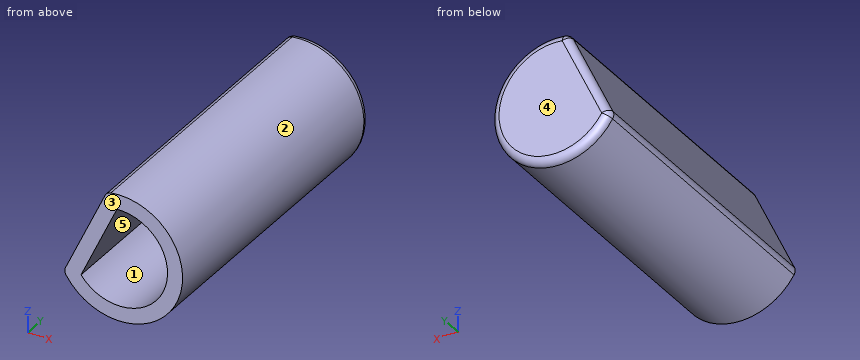
Autodesk Inventor part; units mm, degrees
ref_plane "YZ Plane" through (0, 0, 0) normal (1, 0, 0) x (0, 1, 0)
ref_plane "XZ Plane" through (0, 0, 0) normal (0, 1, 0) x (-1, 0, 0)
ref_plane "XY Plane" through (0, 0, 0) normal (0, 0, 1) x (1, 0, 0)
sketch "Sketch1" plane through (0, 0, 0) normal (0, 1, 0) x (-1, 0, 0)
  arc A0 (0.8395, 4.1153) -> (3.6921, -2.0022) centre (0, 0) ccw
  line L0 (0, -7.6704) -> (0, 6.9519)
  line L1 (-7.5059, 0) -> (5.9652, 0)
  line L2 (3.6921, -2.0022) -> (0.8395, 4.1153)
  dimension "d2" = 8.4
  dimension "d3" = 2.5
  dimension "d4" = 25
extrude "Extrusion1" add sketch "Sketch1" along normal blind 20.4
shell "Shell1" thickness 1 removed faces 1 at (-0.173, 0, 1.1178)
fillet "Fillet1" radius 0.5 2 edges at (-2.2658, 20.4, 1.0565) (3.8065, 20.4, -1.775)
fillet "Fillet2" radius 0.5 4 edges at (-3.5246, 20.2564, -1.9963) (-0.7363, 20.2564, 3.9832) (-0.8395, 9.95, 4.1153) (-3.6921, 9.95, -2.0022)
properties part number "Poti_Verlaengerung"
Can you work these out from the model? Positions are in its coordinate system, mm. Face numbers are marked on the shaded views. A direction names the side the tool comes from. Coordinates: 2 decimals unless noted, no trailing zeros. Loops run counter-clockwise (first coordinate to the right, second up) from the corner with the lowest first, then second, coordinate; pieces in that order, holes last.
Item 1: Please list where these lines run through material, in increasing order: L1, parallel to Z at x = 0, y = 3.75; L2, parallel to Y at x = 1.5, z = 2.5; L3, parallel to Z at x = 1.75, y = 2.5.
Answers below:
L1: z = -4.2 to -3.2, 3.2 to 4.2
L2: y = 19.4 to 20.4
L3: z = -3.82 to -2.68, 2.68 to 3.82
Item 2: Suppose I cut it at A-A (y = 8). Please give me the cut outline in (x, z), then the cut area to 3 significant figures.
Answers below:
outline: (-3.58, -1.76) arc R0.5 ccw to (-3.55, -2.24) arc R4.2 ccw (long way) to (-0.56, 4.16) arc R0.5 ccw to (-0.95, 3.88) - close; hole (-2.55, -1.93) arc R3.2 ccw (long way) to (-0.16, 3.2) - close
area: 22.1 mm2
Item 3: Which directions (+Z, -Z, +X, -X, +Y, -Y) give clear straight access to the entire face, cutting with the end or side of a thin tool? Please do the marked faces 4 and 5.
Answers below:
face 4: +Z, -Z, +X, -X, +Y
face 5: -Y
Item 4: I'm going to push flat-ended pins straight in: pin 1 (1 mm diameter, centred on y = 17.5, z = 2, fed in from -X); pin 2 (1 mm diameter, centred on y = 10.5, z = -1, fed in from +X); pin 3 (1.5 mm diameter, centred on x = 1.5, z = -1.5, fed in from -Y). Where does each tip first touch, or does it pass through?
Answers below:
pin 1: stops at x = -2.06
pin 2: stops at x = 4.17
pin 3: stops at y = 19.4
Item 5: If we mould it in two halves opening along X, with no side actions, what happens to the marked faces 1, 2 and 3? For each: released by +X, released by -X, zero draft, split by the parting line, or undercut.
Answers below:
face 1: undercut
face 2: split by the parting line
face 3: zero draft
